Can you work these out from the model? Positions are in its coordinate system, mm. Face numbers are marked on the shaded views. A direction names the side the tool comes from. Coordinates: 2 decimals unless noted, no trailing zeros. Loops run counter-clockwise (first coordinate to the right, second up) from the corner with the lowest first, then second, coordinate; pieces in that order, holes last.
```python
from build123d import *

# Parameters (mm, degrees)
BOSS_EXTRUDE1_DEPTH = 10.5
FILLET3_R           = 2
SKETCH3_W           = 12.4
SKETCH3_H           = 4.5
SKETCH3_W_2         = 11.854567875
SKETCH3_H_2         = 1.988610451
BOSS_EXTRUDE2_DEPTH = 14.8
SKETCH4_W           = 2
SKETCH4_H           = 2.45
CUT_EXTRUDE1_DEPTH  = 1


with BuildPart() as part:
    # Sketch1 → Boss-Extrude1 (new body)
    with BuildSketch(Plane(origin=(0, 0, 0), x_dir=(1, 0, 0), z_dir=(0, 1, 0))):
        with BuildLine():
            ThreePointArc((-77.532758891, -19.20955436), (-83.896719922, -16.57351539), (-86.532758891, -10.20955436))
            Line((-86.532758891, -10.20955436), (-86.532758891, -1.20955436))
            ThreePointArc((-86.532758891, -1.20955436), (-83.896719922, 5.154406671), (-77.532758891, 7.79044564))
            Line((-77.532758891, 7.79044564), (-22.663339977, 7.79044564))
            Line((-22.663339977, 7.79044564), (-22.663339977, -19.20955436))
            Line((-22.663339977, -19.20955436), (-77.532758891, -19.20955436))
        make_face()
    extrude(amount=BOSS_EXTRUDE1_DEPTH)

    # Fillet3
    fillet3_edges = [part.edges().sort_by_distance(p)[0] for p in [
        (-50.098049434, 10.5, -7.79044564),
        (-83.896719922, 10.5, -5.154406671),
        (-86.532758891, 10.5, 5.70955436),
        (-83.896719922, 10.5, 16.57351539),
        (-86.532758891, 0, 5.70955436),
        (-83.896719922, 0, -5.154406671),
        (-50.098049434, 0, -7.79044564),
        (-50.098049434, 10.5, 19.20955436),
        (-50.098049434, 0, 19.20955436),
        (-83.896719922, 0, 16.57351539),
    ]]
    fillet(fillet3_edges, radius=FILLET3_R)

    # Sketch3 → Boss-Extrude2 (add)
    with BuildSketch(Plane(origin=(-22.663339977, 0, 0), x_dir=(0, 0, -1), z_dir=(1, 0, 0))):
        with Locations((-5.70955436, 5.25)):
            Rectangle(SKETCH3_W, SKETCH3_H)
        with Locations((-5.717006669, 6.244305225)):
            Rectangle(SKETCH3_W_2, SKETCH3_H_2, mode=Mode.SUBTRACT)
    extrude(amount=BOSS_EXTRUDE2_DEPTH)

    # Sketch4 → Cut-Extrude1 (cut)
    with BuildSketch(Plane(origin=(0, 7.5, 0), x_dir=(1, 0, 0), z_dir=(0, 1, 0))):
        with Locations((-14.913433207, -2.660071761)):
            Rectangle(SKETCH4_W, SKETCH4_H)
        with Locations((-14.913433207, -8.429959353)):
            Rectangle(SKETCH4_W, SKETCH4_H)
    extrude(amount=-CUT_EXTRUDE1_DEPTH, mode=Mode.SUBTRACT)


solid = part.part
```
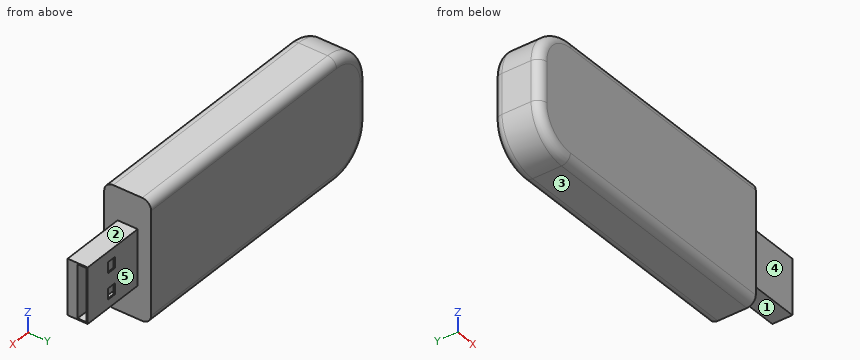
(1) Which directions (+Z, -Z, +X, -X, +Y, -Y) give clear straight access to the entire face, cutting with the end or side of a thin tool? Please do the marked faces 1, 2, 3, 4 and 5.
Check values:
face 1: -Z, +X, +Y, -Y
face 2: +Z, +X, +Y, -Y
face 3: -Z, +X, -X, +Y, -Y
face 4: +Z, -Z, +X, -Y
face 5: +Z, -Z, +X, +Y
(2) If I drill on probe 1 along Z at (x, y) = (-41, 8.75); probe 2 along X at (y, z) = (5.5, 2.75); probe 3 along X at (y, z) = (4.75, 14.5), over which ranges is the centre line in solid material (lowest first)?
Check values:
probe 1: z = -7.77 to 19.19
probe 2: x = -86.53 to -22.66
probe 3: x = -85.44 to -22.66
(3) I want a section at A-A on x = -21.5. Write out the boundary of the cut face in (y, z), then the cut area to 3 significant figures.
Check values:
outline: (3, -0.49) - (7.5, -0.49) - (7.5, 11.91) - (3, 11.91) - close; hole (5.25, -0.21) - (7.24, -0.21) - (7.24, 11.64) - (5.25, 11.64) - close
area: 32.2 mm2
(4) I want a section at C-C on y = 1.25. Write out the boundary of the cut face in (x, z).
Check values:
outline: (-86.39, 1.21) arc R8.85 ccw to (-77.53, -7.64) - (-22.66, -7.64) - (-22.66, 19.06) - (-77.53, 19.06) arc R8.85 ccw to (-86.39, 10.21) - close
(5) I'm going to push flat-ended pins straight in: pin 1 (1 mm diameter, centred on x = -18.5, y = 6.5, fed in from +Z); pin 2 (3.5 mm diameter, centred on x = -12.5, z = 4.5, fed in from -Y); pin 3 (3.5 mm diameter, centred on x = -13.5, y = 6, fed in from -Z). Where does each tip first touch, or does it pass through?
Check values:
pin 1: stops at z = 11.91
pin 2: stops at y = 3
pin 3: stops at z = -0.49
(6) I want a section at B-B on y = 6. Write out the boundary of the cut face in (x, z).
Check values:
outline: (-86.53, 1.21) arc R9 ccw to (-77.53, -7.79) - (-22.66, -7.79) - (-22.66, -0.49) - (-7.86, -0.49) - (-7.86, -0.21) - (-22.66, -0.21) - (-22.66, 11.64) - (-7.86, 11.64) - (-7.86, 11.91) - (-22.66, 11.91) - (-22.66, 19.21) - (-77.53, 19.21) arc R9 ccw to (-86.53, 10.21) - close
